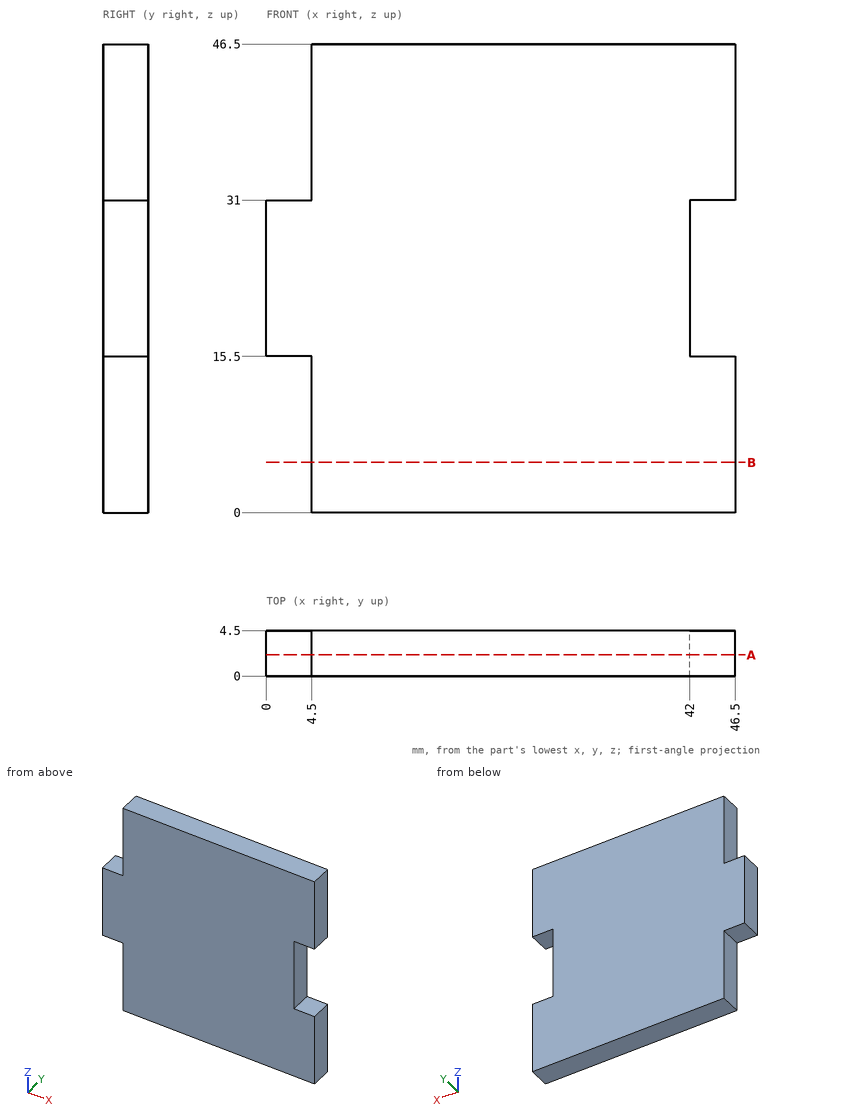
Geometry: see drawing. Coordinates: mm, zero at the bounding-box minimum. Coordinates: 2 decimals unless noted, no trailing zeros. Loops run counter-clockwise (first coordinate to the right, second up) from the corner with the lowest first, then second, coordinate; pieces in that order, holes last. Notation, with made-up numbers: (18, 40) -> (31, 40) arc R6 ccw to (31, 45) -> close; hole circle Ø7 at (-31.5, 56). An arc over 180 degrees is marked (long way). Use a Markdown table: item, result.
1) Contact query for flat-ended pins moving along their axis: pin 1 (1.3 mm diameter, centred on y = 3, z = 4, fed in from -X); pin 2 (2 mm diameter, centred on y = 4, z = 29.5, fed in from +X). Output: stop coordinate, or through.
Results found:
| item | result |
|---|---|
| pin 1 | stops at x = 4.5 |
| pin 2 | stops at x = 42 |
2) Cut plane A-A (y = 2.1). Return the cut outline in (x, z), then the cut area to 3 significant figures.
Results found:
| item | result |
|---|---|
| outline | (0, 15.5) -> (4.5, 15.5) -> (4.5, 0) -> (46.5, 0) -> (46.5, 15.5) -> (42, 15.5) -> (42, 31) -> (46.5, 31) -> (46.5, 46.5) -> (4.5, 46.5) -> (4.5, 31) -> (0, 31) -> close |
| area | 1,950 mm2 |
3) Cut plane B-B (z = 5). Return the cut outline in (x, y).
Results found:
| item | result |
|---|---|
| outline | (4.5, 0) -> (46.5, 0) -> (46.5, 4.5) -> (4.5, 4.5) -> close |
4) Material intervals for line 1 along Z through (x, y) = (42.5, 4.25); line 2 along X through (y, z) = (1.95, 37); line 3 along X through (y, z) = (3.1, 22), sorted ascending. Write a range as from..to.
Results found:
| item | result |
|---|---|
| line 1 | z = 0..15.5, 31..46.5 |
| line 2 | x = 4.5..46.5 |
| line 3 | x = 0..42 |
